For this review, take the finished solid that the model builds, in its own axes (mm). Face numbers are marked on the shaded views. A direction names the side the tool comes from. Coordinates: 2 decimals unless noted, no trailing zeros. Order: outer loops, then holes, each group sorted by start corner. A loop starts at its lowest first (then second) coordinate and runs counter-clockwise, first axis right, second up. Notation, with made-up numbers: (-34, -26) - (-25, -26) arc R25 cw to (-25, -5) - close; hole circle Ø11 at (-13, -33.75). An arc over 180 degrees is marked (long way). One line per item, written item: value. Start each with the question number.
(1) Consider section C-C on z = -12. Write out the cut boundary in (x, y), then the cut area to 3 significant figures.
(2) Consider section B-B on y = 29. Write out the cut boundary in (x, z).
(3) For the marked faces 1 and 2, list the 3-axis set-ups (+Z, -Z, +X, -X, +Y, -Y) from which the entire face can be reached by the end or side of a thin tool; tool diameter is ignored.
(4) To check wall thickness, follow line 1 along X through (y, z) = (36.1, -15.5). State the ranges of the line that lie inside material, in increasing order.
(5) Clearance check with flat-ended pins moving along their axes: pin 1 (1.8 mm diameter, centred on x = -15.5, z = -15.5, fed in from +Y); pin 2 (3.5 mm diameter, centred on x = -15, z = -16, fed in from +Y). State where each tip first meets the part, or that it passes through.
(6) Consider section A-A on z = 0. Write out the cut boundary in (x, y).
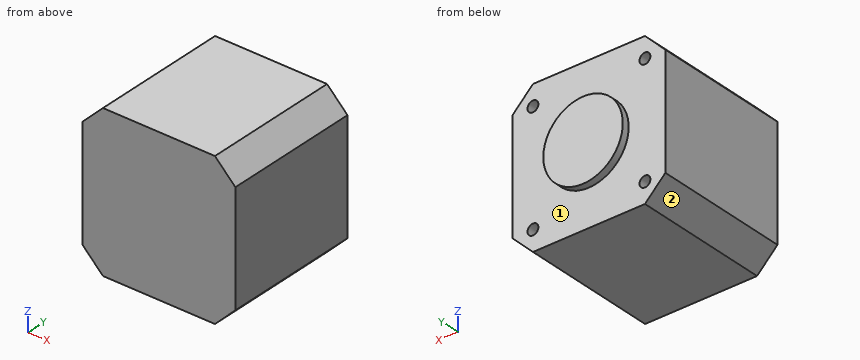
```python
from build123d import *

# Parameters (mm, degrees)
EXTRUDE_1_DEPTH     = 38
SKETCH_3_R          = 11
EXTRUDE_2_DEPTH     = 2
SKETCH_15_R         = 1.5
CUT_EXTRUDE_1_DEPTH = 5


with BuildPart() as part:
    # 草图2 → 凸台-拉伸1 (new body)
    with BuildSketch(Plane(origin=(0, 0, 0), x_dir=(1, 0, 0), z_dir=(0, 1, 0))):
        Polygon((-15.5, 21.15), (-21.15, 15.5), (-21.15, -15.5), (-15.5, -21.15), (15.5, -21.15), (21.15, -15.5), (21.15, 15.5), (15.5, 21.15), align=None)
    extrude(amount=EXTRUDE_1_DEPTH)

    # 草图3 → 凸台-拉伸2 (add)
    with BuildSketch(Plane(origin=(0, 38, 0), x_dir=(1, 0, 0), z_dir=(0, 1, 0))):
        Circle(SKETCH_3_R)
    extrude(amount=EXTRUDE_2_DEPTH)

    # 草图15 → 切除-拉伸1 (cut)
    with BuildSketch(Plane(origin=(0, 38, 0), x_dir=(1, 0, 0), z_dir=(0, 1, 0))):
        with Locations((-15.5, 15.5)):
            Circle(SKETCH_15_R)
        with Locations((15.5, 15.5)):
            Circle(SKETCH_15_R)
        with Locations((15.5, -15.5)):
            Circle(SKETCH_15_R)
        with Locations((-15.5, -15.5)):
            Circle(SKETCH_15_R)
    extrude(amount=-CUT_EXTRUDE_1_DEPTH, mode=Mode.SUBTRACT)


solid = part.part
```
Geometry check:
1. outline: (-21.15, 0) - (21.15, 0) - (21.15, 38) - (-21.15, 38) - close
1. area: 1,610 mm^2
2. outline: (-21.15, -15.5) - (-15.5, -21.15) - (15.5, -21.15) - (21.15, -15.5) - (21.15, 15.5) - (15.5, 21.15) - (-15.5, 21.15) - (-21.15, 15.5) - close
3. face 1: +Y
3. face 2: -Z, -X, +Y, -Y
4. line 1: x = -21.15 to -17, -14 to 14, 17 to 21.15
5. pin 1: stops at y = 33
5. pin 2: stops at y = 38
6. outline: (-21.15, 0) - (21.15, 0) - (21.15, 38) - (11, 38) - (11, 40) - (-11, 40) - (-11, 38) - (-21.15, 38) - close
